The model under review builds one solid part; all positions refer to its coordinate system, in mm. Face numbers are marked on the shaded views. Round coordinates to 2 decimals unless told otherwise and drop trailing zeros. Order: outer loops, then holes, each group sorted by start corner. A loop starts at its lowest first (then second) coordinate and runs counter-clockwise, first axis right, second up.
1) To check wall thickness, follow L1, parallel to X at y = -16.5, z = 10; L2, parallel to Y at x = 10, z = 2.25. State the ranges of each line that lie inside material, in increasing order.
2) Mouldability with a two-part tool opening along X and no side actions: class the marked faces 1, 2 and 3 as pulls with the +X half, pulls with the -X half, needs draft (parallel to the pull), parting line crosses it, or undercut.
3) Consider section B-B (y = -10). Give the boundary of the cut face in (x, z), then the cut area to 3 significant figures.
4) Consider section C-C (y = -2). Give the boundary of the cut face in (x, z).
5) Clearance check with a flat-ended pin moving along its axis: P1, Ø8, axis at y = -10, z = 10, coming from the -X side. State where the tip first meets the part, or that it passes through.
6) Consider section A-A (z = 10). Give the boundary of the cut face in (x, y), then the cut area to 4 significant figures.
7) Consider section D-D (x = 14.5). Give the boundary of the cut face in (y, z).
from build123d import *

# Parameters (mm, degrees)
F0_W     = 20
F0_H     = 20
F1_DEPTH = 20
F3_D     = 10
F5_D     = 10
F7_D     = 10


with BuildPart() as f1:
    # F0 (on Front) → F1 (new body)
    with BuildSketch(Plane.XZ):
        with Locations((10, 10)):
            Rectangle(F0_W, F0_H)
    extrude(amount=F1_DEPTH)

    # F3 (through all)
    with Locations(Plane(origin=(0, 0, 0), x_dir=(1, 0, 0), z_dir=(0, 0, -1))):
        with Locations((10, 10)):
            Hole(F3_D / 2)

    # F5 (through all)
    with Locations(Plane.XZ.offset(20)):
        with Locations((10, 10)):
            Hole(F5_D / 2)

    # F7 (through all)
    with Locations(Plane.YZ.offset(20)):
        with Locations((-10, 10)):
            Hole(F7_D / 2)


solid = f1.part
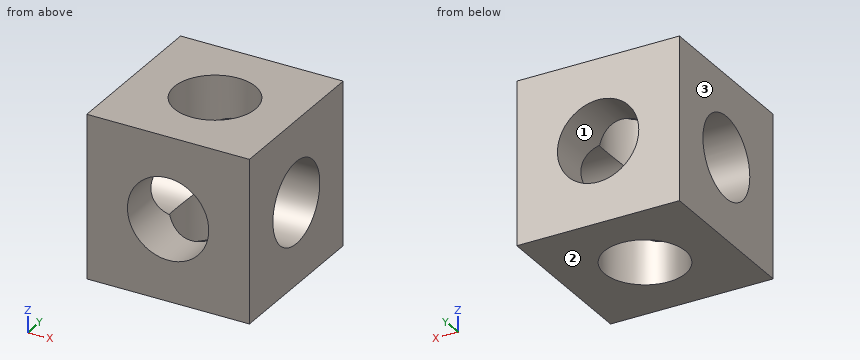
Answer below:
1. L1: x = 0 to 5, 15 to 20
1. L2: y = -20 to -15, -5 to 0
2. face 1: undercut
2. face 2: needs draft
2. face 3: pulls with the -X half
3. outline: (0, 0) - (5, 0) - (5, 5) - (0, 5) - close; (0, 15) - (5, 15) - (5, 20) - (0, 20) - close; (15, 0) - (20, 0) - (20, 5) - (15, 5) - close; (15, 15) - (20, 15) - (20, 20) - (15, 20) - close
3. area: 100 mm2
4. outline: (0, 0) - (20, 0) - (20, 20) - (0, 20) - close; hole circle Ø10 at (10, 10)
5. P1: passes through
6. outline: (0, -20) - (5, -20) - (5, -15) - (0, -15) - close; (0, -5) - (5, -5) - (5, 0) - (0, 0) - close; (15, -20) - (20, -20) - (20, -15) - (15, -15) - close; (15, -5) - (20, -5) - (20, 0) - (15, 0) - close
6. area: 100.0 mm2
7. outline: (-20, 0) - (-12.18, 0) - (-12.18, 5.5) arc R5 cw to (-14.5, 7.82) - (-20, 7.82) - close; (-20, 12.18) - (-14.5, 12.18) arc R5 cw to (-12.18, 14.5) - (-12.18, 20) - (-20, 20) - close; (-7.82, 0) - (0, 0) - (0, 7.82) - (-5.5, 7.82) arc R5 cw to (-7.82, 5.5) - close; (-7.82, 14.5) arc R5 cw to (-5.5, 12.18) - (0, 12.18) - (0, 20) - (-7.82, 20) - close
